```python
from build123d import *

# Parameters (mm, degrees)
SKETCH1_R           = 14.2875
BOSS_EXTRUDE1_DEPTH = 6.35
FILLET2_R           = 101.6
FILLET4_R           = 10.16
FILLET5_R           = 10.16
FILLET6_R           = 10.16
FILLET7_R           = 43.18
FILLET8_R           = 10.16


with BuildPart() as part:
    # Sketch1 → Boss-Extrude1 (new body)
    with BuildSketch(Plane.XY):
        with BuildLine():
            Line((-244.803394078, 23.800923648), (-110.363, 43.529137522))
            Line((-110.363, 43.529137522), (23.636021604, 21.139651339))
            ThreePointArc((23.636021604, 21.139651339), (31.638059922, -2.139986064), (20.574, -24.13))
            Line((20.574, -24.13), (-110.363, -4.730862478))
            Line((-110.363, -4.730862478), (-124.309464555, -6.804936239))
            Line((-124.309464555, -6.804936239), (-127.066874452, 11.985780223))
            Line((-127.066874452, 11.985780223), (-184.996538861, 3.484995791))
            Line((-184.996538861, 3.484995791), (-182.186210881, -15.412181497))
            Line((-182.186210881, -15.412181497), (-241.3, -24.203395818))
            ThreePointArc((-241.3, -24.203395818), (-265.365994979, -1.829751605), (-244.803394078, 23.800923648))
        make_face()
        with Locations((-241.3, -0.073395818)):
            Circle(SKETCH1_R, mode=Mode.SUBTRACT)
        Circle(SKETCH1_R, mode=Mode.SUBTRACT)
    extrude(amount=BOSS_EXTRUDE1_DEPTH)

    # Fillet2
    fillet2_edges = [part.edges().sort_by_distance(p)[0] for p in [
        (-110.363, 43.529137522, 3.175),
    ]]
    fillet(fillet2_edges, radius=FILLET2_R)

    # Fillet4
    fillet4_edges = [part.edges().sort_by_distance(p)[0] for p in [
        (-127.066874452, 11.985780223, 3.175),
    ]]
    fillet(fillet4_edges, radius=FILLET4_R)

    # Fillet5
    fillet5_edges = [part.edges().sort_by_distance(p)[0] for p in [
        (-184.996538861, 3.484995791, 3.175),
    ]]
    fillet(fillet5_edges, radius=FILLET5_R)

    # Fillet6
    fillet6_edges = [part.edges().sort_by_distance(p)[0] for p in [
        (-182.186210881, -15.412181497, 3.175),
    ]]
    fillet(fillet6_edges, radius=FILLET6_R)

    # Fillet7
    fillet7_edges = [part.edges().sort_by_distance(p)[0] for p in [
        (-110.363, -4.730862478, 3.175),
    ]]
    fillet(fillet7_edges, radius=FILLET7_R)

    # Fillet8
    fillet8_edges = [part.edges().sort_by_distance(p)[0] for p in [
        (-124.309464555, -6.804936239, 3.175),
    ]]
    fillet(fillet8_edges, radius=FILLET8_R)


solid = part.part
```
Input: part model. Units: mm. Frame: model coordinates. A direction names the side the tool comes from. Give positions to 0.01 mm unless a question says otherwise; leave off trailing zeros. Write each loop counter-clockwise with the first axis right and the second up, starting at its lowest first coordinate (ties: lowest second). Pieces come first, ordered by that corner, then holes. Notation, with made-up numbers: (74, 75) - (122, 75) arc R25 ccw to (122, 97) - close; hole circle Ø2 at (6, 3). An arc over 180 degrees is marked (long way). Write item = value, one per line. Start each with the question number.
1) Draft query along X for faces 3 (the face through (-155.757, 7.776, 3.131)), 4 (the face through (-115, 10, 0)), 5 (the face through (31.66, -1.79, 3.13)). Return one class per face: pulls with the +X half, pulls with the -X half, needs draft (parallel to the pull), parting line crosses it, or undercut.
2) Material intervals for L1, parallel to X at y = 1.5, z = 5; L2, parallel to Y at x = -241.3, z = 2.5; L3, parallel to Y at x = -252, z = 5, sorted ascending. Write a range as [from, to].
3) Cut plane B-B (z = 4.25). Give the number of separate pieces and of enclosed holes in the cut face, and give its area (3 significant figures).
4) Pin query (flat end, axial travel): pin 1 (2 mm diameter, centred on x = -200.5, y = 33, fed in from +Z); pin 2 (1 mm diameter, centred on y = -4.5, z = 2.5, fed in from -X); pin 3 (3 mm diameter, centred on x = -230.5, z = 5.5, fed in from +Y). Return the tip coordinate at first contact, or that it passes through.
5) Cut plane D-D (y = 18). Return loops of the section in (x, z).
6) Cut plane C-C (x = -80). Return loops of the section in (y, z), and give its area (3 significant figures).
7) Reachability of faces 1 (the face through (-216.4, -20.5, 3.1)), 2 (the face through (-228.102, -5.546, 3.131)) from +Z, -Z, +X, -X, +Y, -Y: full face, straight path, thin tool, end or side. Return the list, or none.
8) Cut plane A-A (x = 0). Return loops of the section in (y, z).
Answers follow:
q1.face_3 = undercut
q1.face_4 = needs draft
q1.face_5 = pulls with the +X half
q2.L1 = [-265.38, -255.5], [-227.1, -181.18], [-125.42, -14.21], [14.21, 31.67]
q2.L2 = [-24.2, -14.36], [14.21, 24.32]
q2.L3 = [-21.7, -9.54], [9.39, 21.55]
q3.separate_pieces = 1
q3.enclosed_holes = 2
q3.area = 11,400 mm^2
q4.pin_1 = through
q4.pin_2 = -265.11
q4.pin_3 = 26.12
q5.outline = (-257.29, 0) - (26.11, 0) - (26.11, 6.35) - (-257.29, 6.35) - close
q6.outline = (-9.23, 0) - (38.46, 0) - (38.46, 6.35) - (-9.23, 6.35) - close
q6.area = 303 mm^2
q7.face_1 = +Z, -Z, -Y
q7.face_2 = +Z, -Z
q8.outline = (-21.08, 0) - (-14.29, 0) - (-14.29, 6.35) - (-21.08, 6.35) - close; (14.29, 0) - (25.09, 0) - (25.09, 6.35) - (14.29, 6.35) - close
